```python
from build123d import *

# Parameters (mm, degrees)
BOSS_EXTRUDE1_DEPTH      = 1.5
BOSS_EXTRUDE1_DEPTH_BACK = 1.5
SKETCH1_R                = 1.6
SKETCH1_R_2              = 2
SKETCH2_R                = 3.025
CUT_EXTRUDE1_DEPTH       = 1
CUT_EXTRUDE2_START       = -1
SKETCH3_R                = 3.025
CUT_EXTRUDE2_DEPTH       = 1
CUT_EXTRUDE3_DEPTH       = 0.75
CUT_EXTRUDE3_DEPTH_BACK  = 0.75
SKETCH4_R                = 1.6
FILLET1_R                = 1
SKETCH5_R                = 1.25
BOSS_EXTRUDE2_DEPTH      = 0.2
BOSS_EXTRUDE3_START      = 0.2
SKETCH6_R                = 1.25
BOSS_EXTRUDE3_DEPTH      = 0.2
CUT_EXTRUDE4_DEPTH       = 1
CUT_EXTRUDE5_START       = -1
CUT_EXTRUDE5_DEPTH       = 1


with BuildPart() as part:
    # Sketch1 → Boss-Extrude1 (new, two sides: drawn at the far end of the back side and taken through both)
    with BuildSketch(Plane(origin=(0, 0, 0), x_dir=(1, 0, 0), z_dir=(0, 1, 0)).offset(-BOSS_EXTRUDE1_DEPTH_BACK)):
        with Locations((0, -6.5)):
            Circle(SKETCH1_R)
        with BuildLine():
            Line((-1.99905303, 6.438461538), (-1.599242424, -6.549230769))
            ThreePointArc((-1.599242424, -6.549230769), (-0.024618299, -4.900189405), (1.6, -6.5))
            ThreePointArc((1.6, -6.5), (1.599810595, -6.524618299), (1.599242424, -6.549230769))
            Line((1.599242424, -6.549230769), (1.99905303, 6.438461538))
            ThreePointArc((1.99905303, 6.438461538), (0, 4.5), (-1.99905303, 6.438461538))
        make_face()
        with Locations((0, 6.5)):
            Circle(SKETCH1_R_2)
    extrude(amount=BOSS_EXTRUDE1_DEPTH + BOSS_EXTRUDE1_DEPTH_BACK)

    # Sketch2 → Cut-Extrude1 (cut)
    with BuildSketch(Plane(origin=(0, 1.5, 0), x_dir=(1, 0, 0), z_dir=(0, 1, 0))):
        with Locations((0, 6.5)):
            Circle(SKETCH2_R)
    extrude(amount=-CUT_EXTRUDE1_DEPTH, mode=Mode.SUBTRACT)

    # Sketch3 → Cut-Extrude2 (cut)
    with BuildSketch(Plane.XZ.offset(1.5).offset(CUT_EXTRUDE2_START)):
        with Locations((0, -6.5)):
            Circle(SKETCH3_R)
    extrude(amount=CUT_EXTRUDE2_DEPTH, mode=Mode.SUBTRACT)

    # Sketch4 → Cut-Extrude3 (cut, two sides: drawn at the far end of the back side and taken through both)
    with BuildSketch(Plane(origin=(0, 0, 0), x_dir=(1, 0, 0), z_dir=(0, 1, 0)).offset(-CUT_EXTRUDE3_DEPTH_BACK)):
        with BuildLine():
            ThreePointArc((-1.6, -6.5), (-1.13137085, -5.36862915), (0, -4.9))
            Line((0, -4.9), (-163.946907064, 159.046907064))
            Line((-163.946907064, 159.046907064), (-163.946907064, -6.5))
            Line((-163.946907064, -6.5), (-1.6, -6.5))
        make_face()
        with BuildLine():
            Line((161.955462973, 157.055462973), (0, -4.9))
            ThreePointArc((0, -4.9), (1.13137085, -5.36862915), (1.6, -6.5))
            Line((1.6, -6.5), (161.955462973, -6.5))
            Line((161.955462973, -6.5), (161.955462973, 157.055462973))
        make_face()
        with BuildLine():
            Line((1.6, -6.5), (0, -6.5))
            Line((0, -6.5), (-1.6, -6.5))
            ThreePointArc((-1.6, -6.5), (0, -8.1), (1.6, -6.5))
        make_face()
        with BuildLine():
            Line((0, -4.9), (0, -6.5))
            Line((0, -6.5), (1.6, -6.5))
            ThreePointArc((1.6, -6.5), (1.13137085, -5.36862915), (0, -4.9))
        make_face()
        with BuildLine():
            Line((-1.6, -6.5), (0, -6.5))
            Line((0, -6.5), (0, -4.9))
            ThreePointArc((0, -4.9), (-1.13137085, -5.36862915), (-1.6, -6.5))
        make_face()
        with Locations((0, -6.5)):
            Circle(SKETCH4_R)
        Polygon((0, -6.5), (-163.946907064, -6.5), (0, -276.849985612), (161.955462973, -6.5), align=None)
    extrude(amount=CUT_EXTRUDE3_DEPTH + CUT_EXTRUDE3_DEPTH_BACK, mode=Mode.SUBTRACT)

    # Fillet1
    fillet1_edges = [part.edges().sort_by_distance(p)[0] for p in [
        (0, 0, 4.9),
    ]]
    fillet(fillet1_edges, radius=FILLET1_R)

    # Sketch5 → Boss-Extrude2 (add)
    with BuildSketch(Plane(origin=(0, 1.5, 0), x_dir=(1, 0, 0), z_dir=(0, 1, 0))):
        with Locations(Location((0, -6.5, 0), (0, 0, 270))):
            Circle(SKETCH5_R)
    extrude(amount=BOSS_EXTRUDE2_DEPTH)

    # Sketch6 → Boss-Extrude3 (add)
    with BuildSketch(Plane.XZ.offset(1.5).offset(BOSS_EXTRUDE3_START)):
        with Locations(Location((0, 6.5, 0), (0, 0, 90))):
            Circle(SKETCH6_R)
    extrude(amount=-BOSS_EXTRUDE3_DEPTH)

    # Sketch7 → Cut-Extrude4 (cut)
    with BuildSketch(Plane(origin=(0, 1.5, 0), x_dir=(1, 0, 0), z_dir=(0, 1, 0))):
        with BuildLine():
            Line((-1.907826404, 3.475), (0, 3.475))
            ThreePointArc((0, 3.475), (-1.025301843, 3.654058832), (-1.929222297, 4.170037268))
            Line((-1.929222297, 4.170037268), (-1.907826404, 3.475))
        make_face()
    extrude(amount=-CUT_EXTRUDE4_DEPTH, mode=Mode.SUBTRACT)

    # Sketch8 → Cut-Extrude5 (cut)
    with BuildSketch(Plane.XZ.offset(1.5).offset(CUT_EXTRUDE5_START)):
        with BuildLine():
            ThreePointArc((-1.929222297, -4.170037268), (-1.025301843, -3.654058832), (0, -3.475))
            Line((0, -3.475), (-1.907826404, -3.475))
            Line((-1.907826404, -3.475), (-1.929222297, -4.170037268))
        make_face()
    extrude(amount=CUT_EXTRUDE5_DEPTH, mode=Mode.SUBTRACT)


solid = part.part
```
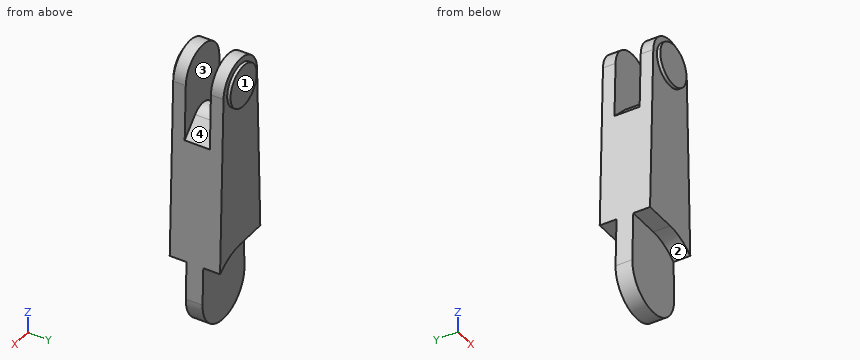
For this review, take the finished solid that the model builds, in its own axes (mm). Face numbers are marked on the shaded views. Round coordinates to 2 decimals unless told otherwise and drop trailing zeros. Loops run counter-clockwise (first coordinate to the right, second up) from the corner with the lowest first, then second, coordinate; pieces in that order, holes last.
Q1. To check wall thickness, follow line 1 along Y through (x, z) = (1.05, 5); line 2 along Z through (x, y) = (-0.1, -1.2) (3 decimals); line 3 along Y through (x, z) = (-1.1, -5.75). State the ranges of each line that lie inside material, in increasing order.
Result sheet:
line 1: y = -1.5 to -0.75, 0.75 to 1.5
line 2: z = -3.475 to 8.097
line 3: y = -0.5 to 0.5
Q2. Insertion check: pin 1 Ø1.5 at (x, y) = (-1.5, 0.5) entering from -Z; pin 2 Ø1.2 at (x, z) = (-0.5, -7) entering from -Y; pin 3 Ø2 at (y, z) = (0, 3.5) entering from +X. Each pin has a flat end and moves straight along its axis. Give the tip position at first contact, or say it passes through.
Result sheet:
pin 1: stops at z = -8.35
pin 2: stops at y = -0.5
pin 3: stops at x = 1.72
Q3. Add section B-B on y = 0.2. Write out the cut boundary in (x, z), plus the area to 3 significant figures.
Result sheet:
outline: (-2, -6.44) arc R2 ccw (long way) to (2, -6.44) - (1.7, 3.2) - (0.71, 4.19) arc R1 ccw to (-0.71, 4.19) - (-1.7, 3.2) - close
area: 44.9 mm2
Q4. Mouldability with a two-part tool opening along Y and no side actions: class the marked faces 1, 2, 3 and 4 as +Y half, -Y half, draft (parallel to the pull), parting line (faces both ways), or undercut.
Result sheet:
face 1: +Y half
face 2: draft
face 3: undercut
face 4: undercut
Q5. Add section A-A on z = 5. Write out the cut boundary in (x, y).
Result sheet:
outline: (-1.65, -1.5) - (1.65, -1.5) - (1.65, -0.75) - (-1.65, -0.75) - close; (-1.65, 0.75) - (1.65, 0.75) - (1.65, 1.5) - (-1.65, 1.5) - close
Q6. Add section D-D on y = -1.15. Write out the cut boundary in (x, z) (3 decimals), plus the area to 3 significant figures.
Result sheet:
outline: (-1.908, -3.475) - (0, -3.475) arc R3.025 cw to (1.929, -4.17) - (1.599, 6.549) arc R1.6 ccw to (-1.599, 6.549) - close
area: 39.4 mm2
Q7. Add section C-C on z = -0.25. Write out the cut boundary in (x, y).
Result sheet:
outline: (-1.81, -1.5) - (1.81, -1.5) - (1.81, 1.5) - (-1.81, 1.5) - close
